Read the model definition and answer for the solid it produces. Units are mm, in the model's axes. Face numbers are marked on the shaded views. A direction names the side the tool comes from. Give positions to 0.01 mm unless a question says otherwise; leave off trailing zeros. Loops run counter-clockwise (first coordinate to the right, second up) from the corner with the lowest first, then second, coordinate; pieces in that order, holes last. Notation, with made-up numbers: (86, 22) -> (95, 22) arc R16 ccw to (95, 42) -> close; hole circle Ø3 at (-39, -3). An arc over 180 degrees is marked (long way). Write each question's results on one line, items separated by ' | '. Start each with the question number.
Item 1: Determine the mould class of the marked faces 1, 2 and 3 for opening direction Z: +Z half, -Z half, draft (parallel to the pull), parting line (faces both ways), or undercut.
Item 2: Section D-D on y = -1 is taken. Write down the section's boundary in (x, z).
Item 3: Section A-A on x = 0 is taken. Write down the section's boundary in (y, z).
Item 4: Find the intervals of material crossed by line 1 (Z direction, x = 4, y = -9); line 2 (Y direction, x = -2, z = 9); line 3 (X direction, y = 2.25, z = 3), in increasing order.
Item 5: Section B-B on y = -5.5 is taken. Write down the section's boundary in (x, z), and give its area (4 significant figures).
Item 6: Each of these flat-tipped pins is pushed along its axis until it touches: P1, Ø2.5, axis at x = 0, y = -4.5, coming from the -Z side; P2, Ø1.2, axis at y = -3.5, z = 9, coming from the +X side; P3, Ø2.5, axis at y = -7, z = -10, coming from the -X side. Where does it stop, or does it pass through?
Item 7: Which of the six approach directions +Z, -Z, +X, -X, +Y, -Y give full straight-line access (tool end or side, diameter ignored) to the marked faces 4, 5, 6, 7 and 8?
Item 8: Section C-C on z = -16 is taken. Write down the section's boundary in (x, y), and give its area (3 significant figures).
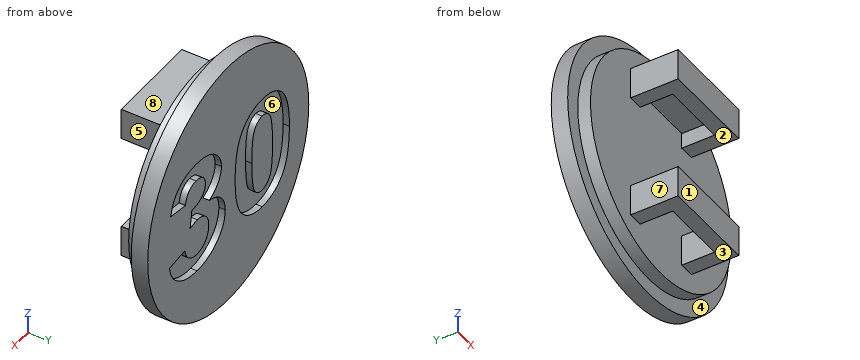
Autodesk Inventor part; units mm, degrees
ref_plane "Work Plane1" through (7.5, -9.5, 10) normal (0, 0, 1) x (1, 0, 0)
ref_plane "YZ Plane" through (0, 0, 0) normal (1, 0, 0) x (0, 1, 0)
ref_plane "XZ Plane" through (0, 0, 0) normal (0, 1, 0) x (-1, 0, 0)
sketch "Sketch1" plane through (0, 0, 0) normal (0, 1, 0) x (-1, 0, 0)
  circle A0 centre (0, 0) radius 19.9
  dimension "d0" = 39.8
extrude "Extrusion1" add sketch "Sketch1" along normal blind 2.6
sketch "Sketch2" plane through (0, 0, 0) normal (0, -1, 0) x (1, 0, 0)
  circle A0 centre (0, 0) radius 19.9
  circle A1 centre (0, 0) radius 17.4
  dimension "d3" = 34.8
extrude "Extrusion2" add sketch "Sketch2" along normal blind 2 contours A1
sketch "Sketch3" plane through (0, -2, 0) normal (0, -1, 0) x (1, 0, 0)
  circle A0 centre (0, 0) radius 17.4
  line L0 (0, 0) -> (0, 17.4) construction
  line L1 (0, 0) -> (17.4, 0) construction
  line L2 (0, 12.5) -> (7.5, 12.5)
  line L3 (7.5, 12.5) -> (7.5, 7.5)
  line L4 (7.5, 7.5) -> (0, 7.5)
  line L5 (0, 12.5) -> (-7.5, 12.5)
  line L6 (-7.5, 12.5) -> (-7.5, 7.5)
  line L7 (-7.5, 7.5) -> (0, 7.5)
  line L8 (0, -12.5) -> (7.5, -12.5)
  line L9 (7.5, -12.5) -> (7.5, -7.5)
  line L10 (7.5, -7.5) -> (0, -7.5)
  line L11 (-7.5, -7.5) -> (0, -7.5)
  line L12 (-7.5, -12.5) -> (-7.5, -7.5)
  line L13 (0, -12.5) -> (-7.5, -12.5)
  dimension "d6" = 15
  dimension "d7" = 5
  dimension "d8" = 15
extrude "Extrusion3" add sketch "Sketch3" along normal blind 7.5 contours L2 L3 L4 L7 L6 L5 | L13 L12 L11 L10 L9 L8
ref_plane "Work Plane1" through (7.5, -9.5, 10) normal (0, 0, 1) x (1, 0, 0)
sketch "Sketch4" plane through (7.5, -2, -12.5) normal (0, 0, -1) x (-1, 0, 0)
  line L0 (0, 0) -> (15, 0)
  line L1 (0, 0) -> (0, -7.5)
  line L2 (15, -7.5) -> (0, -7.5)
  line L3 (15, 0) -> (15, -7.5)
  line L4 (2.35, 0) -> (2.35, -5.15)
  line L5 (2.35, -5.15) -> (12.65, -5.15)
  line L6 (12.65, -5.15) -> (12.65, 0)
  line L7 (2.35, -5.15) -> (0, -5.15) construction
  line L8 (2.35, -5.15) -> (2.35, -7.5) construction
  line L9 (12.65, -5.15) -> (15, -5.15) construction
  point P0 (7.5, 2)
  dimension "d11" = 10.3
extrude "Extrusion4" cut sketch "Sketch4" against normal up to surface (22.5 mm away) contours L0 L6 L5 L4
sketch "Sketch5" plane through (0, 2.6, 0) normal (0, 1, 0) x (1, 0, 0)
  line L0 (15.5957, -8.6476) -> (-15.5957, -8.6476) construction
  line L1 (-15.5957, -8.6476) -> (-15.5957, 11.0665) construction
  line L2 (-15.5957, 11.0665) -> (15.5957, 11.0665) construction
  line L3 (15.5957, 11.0665) -> (15.5957, -8.6476) construction
  line L4 (14.5154, 4.6525) -> (10.6853, 4.2456)
  spline S0 degree 2 poles (10.6853, 4.2456) (10.531, 5.5083) (8.8755, 6.8551) (7.7391, 6.8551) knots 0 0 0 1 2 2 2
  spline S1 degree 2 poles (7.7391, 6.8551) (6.5185, 6.8551) (4.8209, 5.2558) (4.8209, 3.8528) knots 0 0 0 1 2 2 2
  spline S2 degree 2 poles (4.8209, 3.8528) (4.8209, 2.548) (6.4483, 1.0469) (7.6128, 1.0469) knots 0 0 0 1 2 2 2
  spline S3 degree 2 poles (7.6128, 1.0469) (8.3704, 1.0469) (9.4226, 1.2994) knots 0 0 0 1 1 1
  line L5 (9.4226, 1.2994) -> (8.9877, -1.5065)
  spline S4 degree 2 poles (8.9877, -1.5065) (7.4444, -1.4785) (6.5465, -2.0958) knots 0 0 0 1 1 1
  spline S5 degree 2 poles (6.5465, -2.0958) (5.6627, -2.7131) (5.6627, -3.8214) knots 0 0 0 1 1 1
  spline S6 degree 2 poles (5.6627, -3.8214) (5.6627, -4.7614) (6.9534, -5.8136) (7.9495, -5.8136) knots 0 0 0 1 2 2 2
  spline S7 degree 2 poles (7.9495, -5.8136) (8.9596, -5.8136) (10.4328, -4.593) (10.573, -3.4005) knots 0 0 0 1 2 2 2
  line L6 (10.573, -3.4005) -> (14.2348, -3.9477)
  spline S8 degree 2 poles (14.2348, -3.9477) (13.6596, -6.4169) (10.3486, -8.6476) (7.8373, -8.6476) knots 0 0 0 1 2 2 2
  spline S9 degree 2 poles (7.8373, -8.6476) (5.0033, -8.6476) (1.6783, -5.7715) (1.6783, -4.0318) knots 0 0 0 1 2 2 2
  spline S10 degree 2 poles (1.6783, -4.0318) (1.6783, -2.8534) (3.1654, -0.9594) (4.6666, -0.2579) knots 0 0 0 1 2 2 2
  spline S11 degree 2 poles (4.6666, -0.2579) (2.9269, 0.0788) (0.7523, 2.3376) (0.7523, 4.0212) knots 0 0 0 1 2 2 2
  spline S12 degree 2 poles (0.7523, 4.0212) (0.7523, 6.4904) (4.863, 9.7172) (7.711, 9.7172) knots 0 0 0 1 2 2 2
  spline S13 degree 2 poles (7.711, 9.7172) (10.4328, 9.7172) (14.2067, 6.9954) (14.5154, 4.6525) knots 0 0 0 1 2 2 2
  spline S14 degree 2 poles (-8.395, -8.6476) (-11.3973, -8.6476) (-15.1152, -4.565) (-15.1152, 0.5418) knots 0 0 0 1 2 2 2
  spline S15 degree 2 poles (-15.1152, 0.5418) (-15.1152, 5.6346) (-11.3973, 9.7172) (-8.409, 9.7172) knots 0 0 0 1 2 2 2
  spline S16 degree 2 poles (-8.409, 9.7172) (-5.4067, 9.7172) (-1.6888, 5.6626) (-1.6888, 0.4997) knots 0 0 0 1 2 2 2
  spline S17 degree 2 poles (-1.6888, 0.4997) (-1.6888, -4.565) (-5.4067, -8.6476) (-8.395, -8.6476) knots 0 0 0 1 2 2 2
  spline S18 degree 2 poles (-8.395, -5.7855) (-7.2165, -5.7855) (-5.8276, -3.5829) (-5.8276, 0.5418) knots 0 0 0 1 2 2 2
  spline S19 degree 2 poles (-5.8276, 0.5418) (-5.8276, 4.6665) (-7.2165, 6.8551) (-8.395, 6.8551) knots 0 0 0 1 2 2 2
  spline S20 degree 2 poles (-8.395, 6.8551) (-9.5735, 6.8551) (-10.9484, 4.6525) (-10.9484, 0.5418) knots 0 0 0 1 2 2 2
  spline S21 degree 2 poles (-10.9484, 0.5418) (-10.9484, -3.5829) (-9.5735, -5.7855) (-8.395, -5.7855) knots 0 0 0 1 2 2 2
extrude "Extrusion5" cut sketch "Sketch5" against normal blind 1
properties part number "Inside"
Findings:
1) face 1: draft | face 2: undercut | face 3: -Z half
2) outline: circle Ø34.8 at (0, 0)
3) outline: (-9.5, -12.5) -> (-7.15, -12.5) -> (-7.15, -7.5) -> (-9.5, -7.5) -> close; (-9.5, 7.5) -> (-7.15, 7.5) -> (-7.15, 10) -> (-2, 10) -> (-2, -17.4) -> (0, -17.4) -> (0, -19.9) -> (2.6, -19.9) -> (2.6, 19.9) -> (0, 19.9) -> (0, 17.4) -> (-2, 17.4) -> (-2, 12.5) -> (-9.5, 12.5) -> close
4) line 1: -12.5 to -7.5, 7.5 to 12.5 | line 2: -9.5 to -7.15, -2 to 2.6 | line 3: -19.67 to -14.83, -10.75 to -6.03, -1.97 to 1.83, 5.81 to 19.67
5) outline: (-7.5, -12.5) -> (-5.15, -12.5) -> (-5.15, -7.5) -> (-7.5, -7.5) -> close; (-7.5, 7.5) -> (-5.15, 7.5) -> (-5.15, 10) -> (5.15, 10) -> (5.15, 7.5) -> (7.5, 7.5) -> (7.5, 12.5) -> (-7.5, 12.5) -> close; (5.15, -12.5) -> (7.5, -12.5) -> (7.5, -7.5) -> (5.15, -7.5) -> close | area: 72.75 mm2
6) P1: z = 10 | P2: x = 7.5 | P3: x = -7.5
7) face 4: -Y | face 5: +Z, -Z, +X, -Y | face 6: +Y | face 7: +Z, -Z, -X, -Y | face 8: +Z, +X, -X, -Y
8) outline: (-11.83, 0) -> (-6.84, 0) -> (-6.84, -2) -> (6.84, -2) -> (6.84, 0) -> (11.83, 0) -> (11.83, 2.6) -> (-11.83, 2.6) -> close | area: 88.9 mm2
